```python
from build123d import *

# Parameters (mm, degrees)
SKETCH_1_W               = 91
SKETCH_1_H               = 59
EXTRUDE_1_DEPTH          = 3.2
CUT_EXTRUDE_1_DEPTH      = 109.499953917
CUT_EXTRUDE_1_DEPTH_BACK = 109.499953917
CUT_EXTRUDE_2_DEPTH      = 109.499953917
CUT_EXTRUDE_2_DEPTH_BACK = 109.499953917
SKETCH_3_R               = 2.067


with BuildPart() as part:
    # ｽｹｯﾁ1 → ﾎﾞｽ - 押し出し1 (new body)
    with BuildSketch(Plane.XY):
        with Locations((45.5, 29.5)):
            Rectangle(SKETCH_1_W, SKETCH_1_H)
    extrude(amount=EXTRUDE_1_DEPTH)

    # ｽｹｯﾁ2 → ｶｯﾄ - 押し出し1 (cut, two sides: drawn at the far end of the back side and taken through both)
    with BuildSketch(Plane.XY.offset(-CUT_EXTRUDE_1_DEPTH_BACK)):
        with BuildLine():
            Line((11, 51.5), (81, 51.5))
            ThreePointArc((81, 51.5), (84.5, 48), (81, 44.5))
            Line((81, 44.5), (11, 44.5))
            ThreePointArc((11, 44.5), (7.5, 48), (11, 51.5))
        make_face()
    extrude(amount=CUT_EXTRUDE_1_DEPTH + CUT_EXTRUDE_1_DEPTH_BACK, mode=Mode.SUBTRACT)

    # ｽｹｯﾁ3 → ｶｯﾄ - 押し出し2 (cut, two sides: drawn at the far end of the back side and taken through both)
    with BuildSketch(Plane.XY.offset(-CUT_EXTRUDE_2_DEPTH_BACK)):
        with Locations((72, 35)):
            Circle(SKETCH_3_R)
        with Locations((72, 4.8)):
            Circle(SKETCH_3_R)
    extrude(amount=CUT_EXTRUDE_2_DEPTH + CUT_EXTRUDE_2_DEPTH_BACK, mode=Mode.SUBTRACT)


solid = part.part
```
The model under review builds one solid part; all positions refer to its coordinate system, in mm. A direction names the side the tool comes from. Round coordinates to 2 decimals unless told otherwise and drop trailing zeros. Order: outer loops, then holes, each group sorted by start corner. A loop starts at its lowest first (then second) coordinate and runs counter-clockwise, first axis right, second up.
Item 1: Machinability: for faces 4 (the flat face through (45, 30, 3.2)), 5 (the flat face through (46, 51.5, 2)), which of the approach directions +Z, -Z, +X, -X, +Y, -Y give a long, thin tool a straight path to every point of the face, cutting with its end or side? Answer none if there is none.
Working result:
face 4: +Z, +X, -X, +Y, -Y
face 5: +Z, -Z
Item 2: Add section C-C, the plane z = 2.15. State the section outline as (x, y) points, and give its area (3 significant figures).
Working result:
outline: (0, 0) - (91, 0) - (91, 59) - (0, 59) - close; hole (11, 44.5) - (81, 44.5) arc R3.5 ccw to (81, 51.5) - (11, 51.5) arc R3.5 ccw to start; hole circle Ø4.13 at (72, 4.8); hole circle Ø4.13 at (72, 35)
area: 4,810 mm2
Item 3: Add section A-A, the plane y = 48. State the section outline as (x, z) points.
Working result:
outline: (0, 0) - (7.5, 0) - (7.5, 3.2) - (0, 3.2) - close; (84.5, 0) - (91, 0) - (91, 3.2) - (84.5, 3.2) - close
Item 4: Draft analysis for pull direction Y (two halves, no side actions). For faces 1 (the flat face through (45, 59, 2)), 2 (the cylindrical face through (7.5, 47.9, 1.6)), 3 (the flat face through (45, 30, 0)), state which applies: released by +Y, released by -Y, zero draft, split by the parting line, or undercut.
Working result:
face 1: released by +Y
face 2: undercut
face 3: zero draft
Item 5: Add section B-B, the plane x = 78. State the section outline as (y, z) points, and give its area (3 significant figures).
Working result:
outline: (0, 0) - (44.5, 0) - (44.5, 3.2) - (0, 3.2) - close; (51.5, 0) - (59, 0) - (59, 3.2) - (51.5, 3.2) - close
area: 166 mm2
Item 6: To check wall thickness, follow probe 1 along Y at (x, z) = (72, 2.25); probe 2 along X at (y, z) = (4.8, 2.5); probe 3 along Y at (x, z) = (68.5, 3.05). State the ranges of each line that lie inside material, in increasing order.
Working result:
probe 1: y = 0 to 2.73, 6.87 to 32.93, 37.07 to 44.5, 51.5 to 59
probe 2: x = 0 to 69.93, 74.07 to 91
probe 3: y = 0 to 44.5, 51.5 to 59
Item 7: For pin 1 (1 mm diameter, centred on x = 43, z = 2, fed in from -Y), flat-tipped, find the tip position at first contact; note if it passes through.
Working result:
pin 1: stops at y = 0
